from build123d import *

# Parameters (mm, degrees)
F0_R     = 25.4
F0_R_2   = 6.35
F0_R_3   = 4.445
F1_DEPTH = 25.4
F3_SIZE  = 5.08


# Not quite as in the source:
# - a fillet or chamfer that OpenCascade refuses, or shapes differently, is made with other operations: its cross-section is extruded or revolved along the edge and cut away or added


with BuildPart() as f1:
    # F0 (on Top) → F1 (new body)
    with BuildSketch(Plane.XY):
        Circle(F0_R)
        Circle(F0_R_2, mode=Mode.SUBTRACT)
        with Locations((0, 19.05)):
            Circle(F0_R_3, mode=Mode.SUBTRACT)
    extrude(amount=F1_DEPTH)

    # F2: fillet of radius 5.08 on 1 edges, made by hand

    # F2_s1 → F2_t2 (revolve, cut)
    with BuildSketch(Plane.XZ):
        with BuildLine():
            ThreePointArc((25.4, 20.32), (23.9121024484, 23.9121024484), (20.32, 25.4))
            Line((20.32, 25.4), (25.4, 25.4))
            Line((25.4, 25.4), (25.4, 20.32))
        make_face()
    revolve(axis=Axis((0, 0, 25.4), (0, 0, 1)), mode=Mode.SUBTRACT)

    # F3
    f3_edges = [f1.edges().sort_by_distance(p)[0] for p in [
        (-6.35, 0, 25.4),
    ]]
    chamfer(f3_edges, length=F3_SIZE)


solid = f1.part
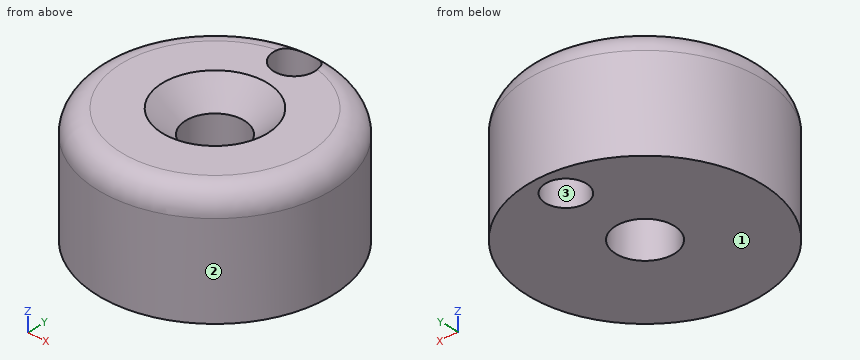
Can you work these out from the model? Positions are in its coordinate system, mm. Face numbers are marked on the shaded views. Coordinates: 2 decimals unless noted, no trailing zeros. Write each loop counter-clockwise with the first axis right and the second up, starting at its lowest first coordinate (ties: lowest second). Pieces come first, ordered by that corner, then holes. Notation, with made-up numbers: (-38.75, 14.5) -> (-24.75, 14.5) arc R19 cw to (-24.75, 39.5) -> close; hole circle Ø8 at (22, -24). An arc over 180 degrees is marked (long way). Write each question's results on one line, items separated by ' | '. Start each with the question number.
Q1. We'd pull the mould along X, two halves only. Please class the marked faces 1, 2 and 3: +X half, -X half, draft (parallel to the pull), parting line (faces both ways), or undercut.
Q2. I'm going to push flat-ended pins straight in: pin 1 (2 mm diameter, centred on y = 19.5, z = 11.5, fed in from +X); pin 2 (5 mm diameter, centred on x = 10, z = 4, fed in from -Y); pin 3 (3 mm diameter, centred on y = 17, z = 19, fed in from -X). Where does each tip first touch, or does it pass through?
Q3. Imagine slicing it at A-A (x = 0). Write out the boundary of the cut face in (y, z) (3 decimals), then the cut area to 3 significant figures.
Q4. If I drill on probe 1 along Y at (x, z) = (0, 11.25) (3 decimals); probe 2 along Y at (x, z) = (-2, 18.75); probe 3 along X at (y, z) = (19.05, 10) (3 decimals), over which ranges is the centre line in solid material (lowest first)?
Q5. Imagine slicing it at B-B (z = 15.25). Write out the boundary of the cut face in (x, y) (3 decimals).
Taken from the geometry:
1) face 1: draft | face 2: parting line | face 3: undercut
2) pin 1: stops at x = 17.4 | pin 2: stops at y = -24.27 | pin 3: stops at x = -20.12
3) outline: (-25.4, 0) -> (-6.35, 0) -> (-6.35, 20.32) -> (-11.43, 25.4) -> (-20.32, 25.4) arc R5.08 ccw to (-25.4, 20.32) -> close; (6.35, 0) -> (14.605, 0) -> (14.605, 25.4) -> (11.43, 25.4) -> (6.35, 20.32) -> close; (23.495, 0) -> (25.4, 0) -> (25.4, 20.32) arc R5.08 ccw to (23.495, 24.286) -> close | area: 706 mm^2
4) probe 1: y = -25.4 to -6.35, 6.35 to 14.605, 23.495 to 25.4 | probe 2: y = -25.32 to -6.03, 6.03 to 15.08, 23.02 to 25.32 | probe 3: x = -16.801 to -4.445, 4.445 to 16.801
5) outline: circle Ø50.8 at (0, 0); hole circle Ø12.7 at (0, 0); hole circle Ø8.89 at (0, 19.05)
